Source: three-view drawing plus pictorial views. Frame: mm from the lowest corner of the part. A direction names the side the tool comes from. Coordinates: 2 decimals unless noted, no trailing zeros. Loops run counter-clockwise (first coordinate to the right, second up) from the corner with the lowest first, then second, coordinate; pieces in that order, holes last. Notation, with made-up numbers: (9, -38.5) -> (17, -38.5) arc R15 ccw to (17, -25.5) -> close; hole circle Ø6 at (0.25, -9.5). An arc over 180 degrees is marked (long way). Answer as a JSON object with one key per item and string values. Group by question number.
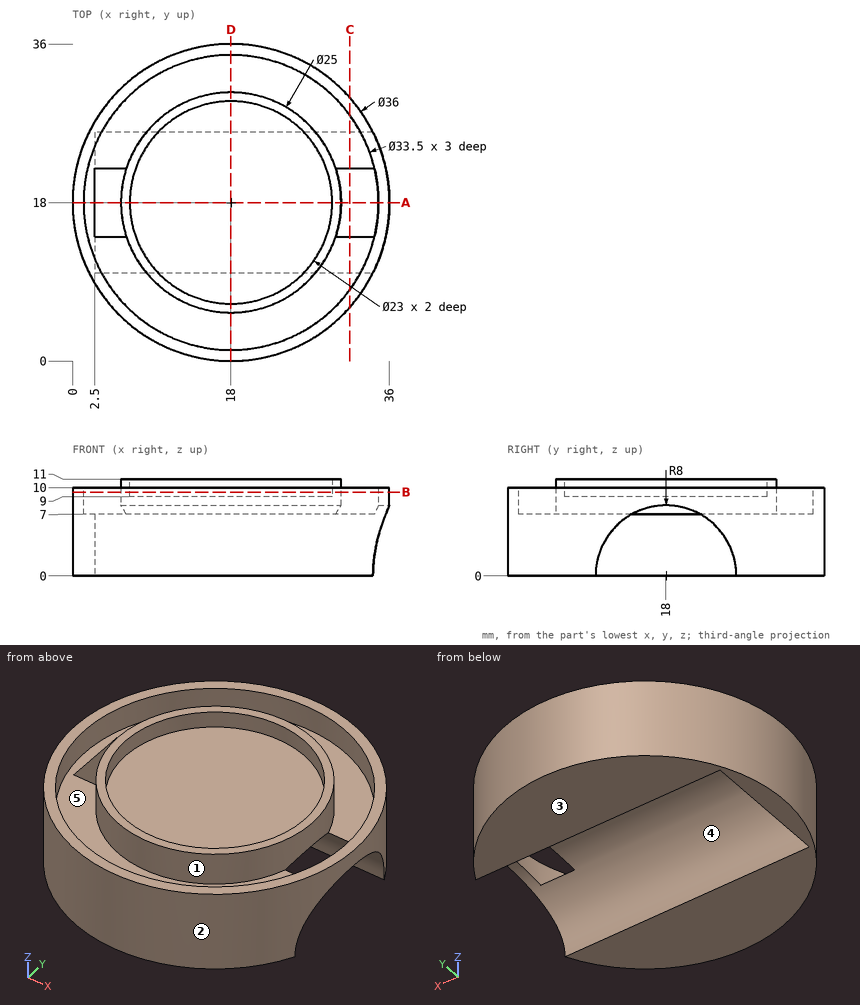
1. Reachability of the marked faces 4 and 5 from +Z, -Z, +X, -X, +Y, -Y: full face, straight path, thin tool, end or side. Return the list, or none.
2. Section query A-A on y = 18. Return loops of the section in (x, z).
3. Section query D-D on x = 18. Return loops of the section in (y, z).
4. Ray query, L1, parallel to Y at x = 18, z = 10.5; L2, parallel to Y at x = 23, z = 8.25; L3, parallel to Z at x = 11.5, y = 18. Return the intervals inside material, ascending.
5. Mould query, pull axis X, two halves, no side actions, for the marked faces 1, 2 and 3. Classes: pulls with the +X half, pulls with the -X half, needs draft (parallel to the pull), parting line crosses it, or undercut.
6. Pin query (flat end, axial travel): pin 1 Ø11 at (x, y) = (18.5, 16) entering from +Z; pin 2 Ø2 at (x, z) = (27.5, 6.5) entering from -Y; pin 3 Ø1.5 at (x, z) = (24, 2.5) entering from -Y. Return the tip coordinate at first contact, or that it passes through.
7. Section query B-B on z = 9.5. Return loops of the section in (x, y).
8. Section query C-C on x = 31.5. Return loops of the section in (y, z), then the cut area to 3 significant figures.
Solved:
{
 "1": {"face 4": "-Z, +X", "face 5": "+Z"},
 "2": {"outline": "(0, 0) -> (2.5, 0) -> (2.5, 7) -> (1.25, 7) -> (1.25, 10) -> (0, 10) -> close; (5.5, 8) -> (30.5, 8) -> (30.5, 11) -> (29.5, 11) -> (29.5, 9) -> (6.5, 9) -> (6.5, 11) -> (5.5, 11) -> close; (34.75, 8) -> (36, 8) -> (36, 10) -> (34.75, 10) -> close"},
 "3": {"outline": "(0, 0) -> (10, 0) arc R8 cw to (26, 0) -> (36, 0) -> (36, 10) -> (34.75, 10) -> (34.75, 7) -> (30.5, 7) -> (30.5, 11) -> (29.5, 11) -> (29.5, 9) -> (6.5, 9) -> (6.5, 11) -> (5.5, 11) -> (5.5, 7) -> (1.25, 7) -> (1.25, 10) -> (0, 10) -> close"},
 "4": {"L1": "5.5 to 6.5, 29.5 to 30.5", "L2": "0.71 to 2.01, 6.54 to 29.46, 33.99 to 35.29", "L3": "8 to 9"},
 "5": {"face 1": "undercut", "face 2": "parting line crosses it", "face 3": "needs draft"},
 "6": {"pin 1": "z = 9", "pin 2": "y = 2.13", "pin 3": "y = 0.78"},
 "7": {"outline": "circle Ø36 at (18, 18); circle Ø25 at (18, 18); hole circle Ø33.5 at (18, 18); hole circle Ø23 at (18, 18)"},
 "8": {"outline": "(6.09, 0) -> (10, 0) arc R8 cw to (14.13, 7) -> (8.08, 7) -> (8.08, 10) -> (6.09, 10) -> close; (21.87, 7) arc R8 cw to (26, 0) -> (29.91, 0) -> (29.91, 10) -> (27.92, 10) -> (27.92, 7) -> close", "area": "83.3 mm^2"}
}
